Build history of the part. All positions in model axes, mm. A direction names the side the tool comes from. Round coordinates to 2 decimals unless told otherwise and drop trailing zeros. Loops run counter-clockwise (first coordinate to the right, second up) from the corner with the lowest first, then second, coordinate; pieces in that order, holes last. Notation, with made-up numbers: (-15, 17.5) - (36, 17.5) arc R14 ccw to (36, 30.5) - close; hole circle Ø3 at (8, 64). An arc over 180 degrees is marked (long way). Use one line per item in the form item = value. Start each with the question number.
Q1. Pin check, flat tips, straight feed: pin 1 (1.5 mm diameter, centred on y = 77.5, z = -2.5, fed in from +X); pin 2 (1 mm diameter, centred on x = 5, z = -1.5, fed in from -Y); pin 3 (6 mm diameter, centred on x = -4.5, y = 70.5, fed in from -Z); pin 4 (1.5 mm diameter, centred on y = 132.5, z = 1, fed in from +X). Stop position of each tip, or through.
Q2. Saw through at A-A (x = 0). Give the cut face in (y, z), then the cut area to 3 significant figures.
Q3. 3-axis set-ups, long thin cutter, end or side, ignore diameter. For faces 1 (the face through (0.78, 68.75, -5.95)), 2 (the face through (0, 136, 5)), 3 (the face through (0, 0, 0)), 4 (the face through (4.75, 7, 0)), 5 (the face through (-4.75, 7, 0)): which of +Z, -Z, +X, -X, +Y, -Y reach the whole face in a straight line?
Q4. Saw through at C-C (y = 99). Give the cut face in (x, z).
Q5. Saw through at B-B (z = 0). Give the cut face in (x, y).
Q6. Drill centre lines: line 1 (Y direction, x = -3, z = -4.5); line 2 (X direction, y = 42.5, z = -0.25); line 3 (Z direction, x = -0.5, y = 121.5). Where is each one in solid material? Low to high.
```python
from build123d import *

# Parameters (mm, degrees)
SKETCH2_W          = 2.5
SKETCH2_H          = 15
CUT_EXTRUDE1_DEPTH = 15
CHAMFER1_SIZE      = 0.4
FILLET1_R          = 0.4


with BuildPart() as part:
    # Sketch1 → Revolve1 (revolve)
    with BuildSketch(Plane.XY):
        Polygon((0, 0), (-6, 0), (-6, 136), (-4, 136), (-4, 150), (0, 150), align=None)
    revolve(axis=Axis((0, 150, 0), (0, -1, 0)))

    # Sketch2 → Cut-Extrude1 (cut, symmetric)
    with BuildSketch(Plane.XY):
        with Locations((-6, 7.5)):
            Rectangle(SKETCH2_W, SKETCH2_H)
    cut_extrude1 = extrude(amount=CUT_EXTRUDE1_DEPTH, both=True, mode=Mode.SUBTRACT)

    # Mirror1: Cut-Extrude1 across plane
    add(cut_extrude1.mirror(Plane(origin=(0, 0, 0), x_dir=(0, 0, 1), z_dir=(1, 0, 0))), mode=Mode.SUBTRACT)

    # Chamfer1
    chamfer1_edges = [part.edges().sort_by_distance(p)[0] for p in [
        (4, 150, 0),
    ]]
    chamfer(chamfer1_edges, length=CHAMFER1_SIZE)

    # Fillet1
    fillet1_edges = [part.edges().sort_by_distance(p)[0] for p in [
        (4, 136, 0),
        (6, 136, 0),
    ]]
    fillet(fillet1_edges, radius=FILLET1_R)


solid = part.part
```
Report:
q1.pin_1 = 5.74
q1.pin_2 = 0
q1.pin_3 = -5.81
q1.pin_4 = 5.99
q2.outline = (0, -6) - (135.6, -6) arc R0.4 ccw to (136, -5.6) - (136, -4.4) arc R0.4 cw to (136.4, -4) - (149.6, -4) - (150, -3.6) - (150, 3.6) - (149.6, 4) - (136.4, 4) arc R0.4 cw to (136, 4.4) - (136, 5.6) arc R0.4 ccw to (135.6, 6) - (0, 6) - close
q2.area = 1,740 mm²
q3.face_1 = +Y, -Y
q3.face_2 = +Y
q3.face_3 = +Z, -Z, +X, -X, -Y
q3.face_4 = +Z, -Z, +X, -Y
q3.face_5 = +Z, -Z, -X, -Y
q4.outline = circle Ø12 at (0, 0)
q5.outline = (-6, 15) - (-4.75, 15) - (-4.75, 0) - (4.75, 0) - (4.75, 15) - (6, 15) - (6, 135.6) arc R0.4 ccw to (5.6, 136) - (4.4, 136) arc R0.4 cw to (4, 136.4) - (4, 149.6) - (3.6, 150) - (-3.6, 150) - (-4, 149.6) - (-4, 136.4) arc R0.4 cw to (-4.4, 136) - (-5.6, 136) arc R0.4 ccw to (-6, 135.6) - close
q6.line_1 = 0 to 136
q6.line_2 = -5.99 to 5.99
q6.line_3 = -5.98 to 5.98
